from build123d import *

# Parameters (mm, degrees)
F1_DEPTH = 12.7
F2_W     = 6.35
F2_H     = 25.4
F3_DEPTH = 12.7
F4_W     = 12.7
F4_H     = 6.35
F5_DEPTH = 25.4


with BuildPart() as f1:
    # F0 (on Top) → F1 (new body)
    with BuildSketch(Plane.XY):
        Polygon((0, 25.4), (0, 0), (38.1, 0), (38.1, 6.35), (23.706993, 6.35), (23.706993, 19.05), (38.1, 19.05), (38.1, 25.4), align=None)
    extrude(amount=F1_DEPTH)

    # F2 (on face) → F3 (join)
    with BuildSketch(Plane.XY.offset(12.7)):
        with Locations((3.175, 12.7)):
            Rectangle(F2_W, F2_H)
    extrude(amount=F3_DEPTH)

    # F4 (on face) → F5 (cut)
    with BuildSketch(Plane.YZ.offset(6.35)):
        with Locations((12.7, 22.225)):
            Rectangle(F4_W, F4_H)
    extrude(amount=-F5_DEPTH, mode=Mode.SUBTRACT)


solid = f1.part
The listing builds one solid part. Answer for the finished solid, in the listing's coordinates (mm). A direction names the side the tool comes from. Give positions to 0.01 mm unless a question says otherwise; leave off trailing zeros. Write each loop counter-clockwise with the first axis right and the second up, starting at its lowest first coordinate (ties: lowest second). Pieces come first, ordered by that corner, then holes.
1) Section B-B (x = 25.5) is taken. Write down the section's boundary in (y, z).
2) Section D-D (z = 12.25) is taken. Write down the section's boundary in (x, y), and give its area (3 significant figures).
3) For a pull along Y with two mould halves and no side action, classify faces 5 (the face through (15, 0, 10)), 6 (the face through (31, 19.05, 6)), 7 (the face through (6.35, 13, 18)), 8 (the face through (23.707, 13, 6)) as pulls with the +Y half, pulls with the -Y half, needs draft (parallel to the pull), parting line crosses it, or undercut.
4) Given P1, Ø12.5, axis at x = 20, y = 8, coming from the +Z side; P2, Ø4, axis at y = 13, z = 9, coming from the +X side, each flat-ended and moving along its own axis, determine where each tip first touches the part or whether it passes through.
5) A tool of negligible diameter and unlimited length cuts with its end or side. For faces 1 (the face through (3, 13, 19.05)), 2 (the face through (18, 13, 12.7)), 3 (the face through (38.1, 3, 6)), 4 (the face through (31, 6.35, 6)), from which of +Z, -Z, +X, -X, +Y, -Y can it reach the whole face along a straight path? Write none if from no direction.
6) Section A-A (z = 20.75) is taken. Write down the section's boundary in (x, y).
7) Section C-C (y = 10.5) is taken. Write down the section's boundary in (x, z).
8) Find the intervals of material crossed by L1, parallel to Y at x = 29, z = 4.5; L2, parallel to Z at x = 20.5, y = 18; L3, parallel to X at y = 3.5, z = 22.75, in increasing order.
Response:
1. outline: (0, 0) - (6.35, 0) - (6.35, 12.7) - (0, 12.7) - close; (19.05, 0) - (25.4, 0) - (25.4, 12.7) - (19.05, 12.7) - close
2. outline: (0, 0) - (38.1, 0) - (38.1, 6.35) - (23.71, 6.35) - (23.71, 19.05) - (38.1, 19.05) - (38.1, 25.4) - (0, 25.4) - close
2. area: 785 mm2
3. face 5: pulls with the -Y half
3. face 6: undercut
3. face 7: needs draft
3. face 8: undercut
4. P1: stops at z = 12.7
4. P2: stops at x = 23.71
5. face 1: +Z, +X, -X
5. face 2: +Z, +X, +Y, -Y
5. face 3: +Z, -Z, +X, +Y, -Y
5. face 4: +Z, -Z, +X
6. outline: (0, 0) - (6.35, 0) - (6.35, 6.35) - (0, 6.35) - close; (0, 19.05) - (6.35, 19.05) - (6.35, 25.4) - (0, 25.4) - close
7. outline: (0, 0) - (23.71, 0) - (23.71, 12.7) - (6.35, 12.7) - (6.35, 19.05) - (0, 19.05) - close
8. L1: y = 0 to 6.35, 19.05 to 25.4
8. L2: z = 0 to 12.7
8. L3: x = 0 to 6.35
